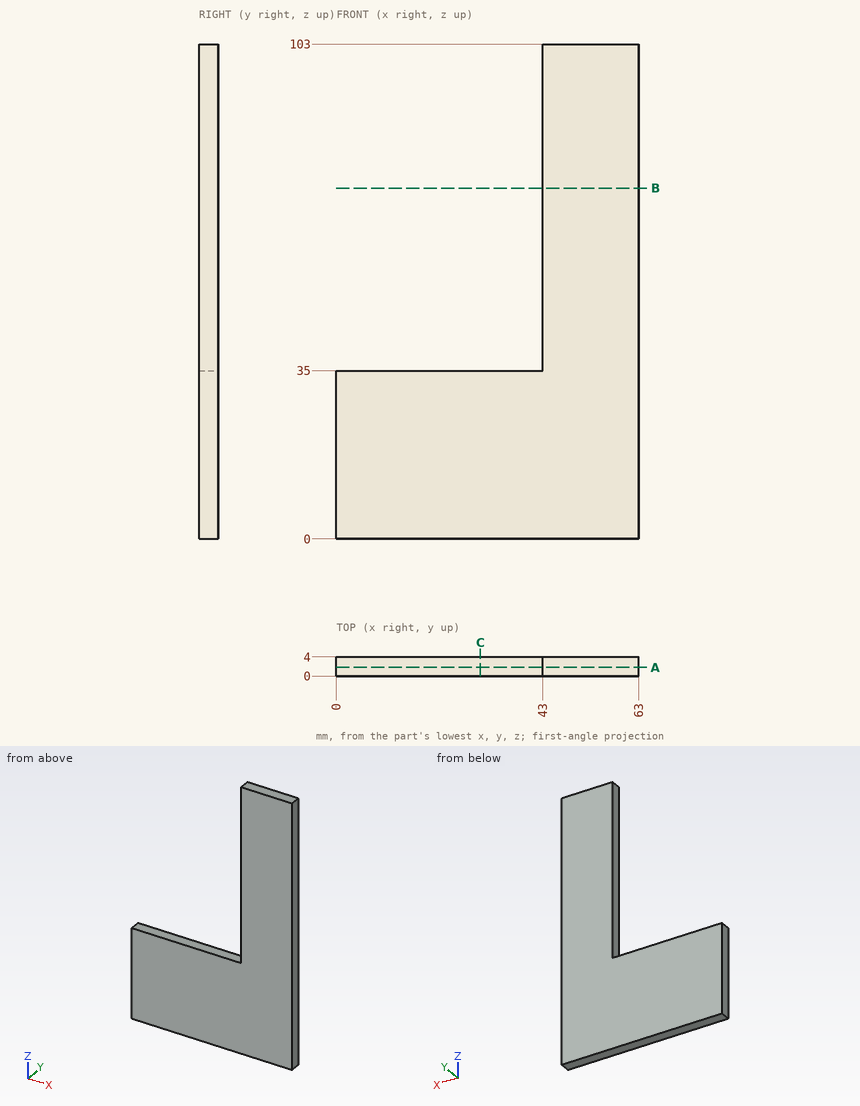
Drawing for the job (mm, zero at the part's lowest x, y, z). Round coordinates to 2 decimals unless told otherwise and drop trailing zeros. Write each loop counter-clockwise with the first axis right and the second up, starting at its lowest first coordinate (ties: lowest second). Pieces come first, ordered by that corner, then holes.
Item 1: Drill centre lines: L1, parallel to Z at x = 23.5, y = 3.1; L2, parallel to X at y = 0.5, z = 78.5. Where is each one in solid material? Low to high.
Filled in:
L1: z = 0 to 35
L2: x = 43 to 63
Item 2: Band-saw the part on A-A on y = 1.8. Write the cut outline in (x, z), then the cut area to 4 significant figures.
Filled in:
outline: (0, 0) - (63, 0) - (63, 103) - (43, 103) - (43, 35) - (0, 35) - close
area: 3,565 mm2
Item 3: Band-saw the part on B-B on z = 73. Write the cut outline in (x, y).
Filled in:
outline: (43, 0) - (63, 0) - (63, 4) - (43, 4) - close
Item 4: Band-saw the part on C-C on x = 30. Write the cut outline in (y, z).
Filled in:
outline: (0, 0) - (4, 0) - (4, 35) - (0, 35) - close
Item 5: Drop a flat-ended pin along its axis: pin 1 Ø1.5 at (y, z) = (3, 57) entering from -X. Give the stop position or say it passes through.
Filled in:
pin 1: stops at x = 43
